Model file for the job. Use its own axes, mm. Face numbers are marked on the shaded views. A direction names the side the tool comes from. Round coordinates to 2 decimals unless told otherwise and drop trailing zeros. Loops run counter-clockwise (first coordinate to the right, second up) from the corner with the lowest first, then second, coordinate; pieces in that order, holes last. Notation, with made-up numbers: M 8.5,-29.75 L 52.5,-29.75 A8 cw 52.5,-19.75 Z; hole C 80.25,54 d4. An arc over 180 degrees is marked long. Use a Markdown table: item, result. Add a question column.
Item 1: Wall check: L1, parallel to Z at x = 6.5, y = -2; L2, parallel to Z at x = 5.25, y = 2.5; L3, parallel to Y at x = 5, z = 0.25. Give the ranges that are in metal, low to high. Write a range as from..to.
Item 2: Saw through at A-A on y = -0.25. Write the cut outline in (x, z), then the cut area to 3 significant figures.
Item 3: Pin check, flat tips, straight feed: P1, Ø0.7, axis at y = 3, z = 3.5, coming from the +X side; P2, Ø0.5, axis at x = 6, z = -5.5, coming from the +Y side; P3, Ø4, axis at y = -3.5, z = 0, coming from the -X side; P4, Ø1.2, axis at x = -6.5, y = -1.5, coming from the +Z side. Stop position of each tip, or through.
Item 4: Saw through at B-B on x = -2.25. Write the cut outline in (y, z).
Item 5: Saw through at C-C on z = -4.25. Write the cut outline in (x, y).
Item 6: Saw through at D-D on y = 2.25. Write the cut outline in (x, z), then the cut area to 3 significant figures.
Item 7: Two-plate mould, pull along X, no slides. Class the marked faces 4, 5 and 6: +X half, -X half, draft (parallel to the pull), parting line (faces both ways), or undercut.
Item 8: Tool access for the marked faces 1, 2 and 3: list every direction of +Z, -Z, +X, -X, +Y, -Y with a clear straight run to the whole face (end or side of a thin tool).
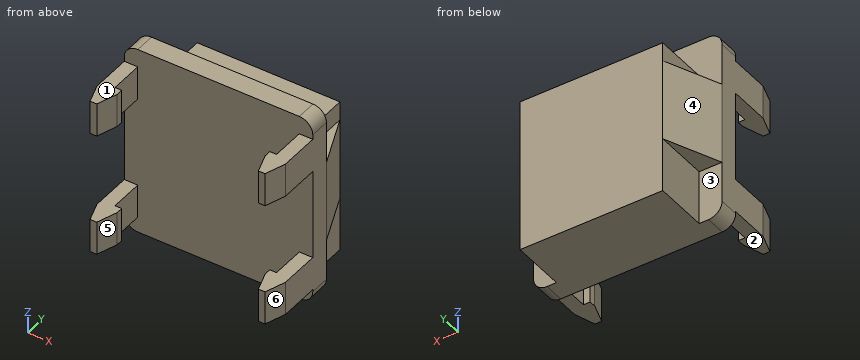
```python
from build123d import *

# Parameters (mm, degrees)
BOSS_EXTRUDE1_DEPTH = 1.5
SKETCH2_W           = 10.6
SKETCH2_H           = 11.5
BOSS_EXTRUDE2_DEPTH = 4
BOSS_EXTRUDE4_DEPTH = 6.07
SKETCH5_W           = 1.5
SKETCH5_H           = 2.5
BOSS_EXTRUDE5_DEPTH = 4.5
SKETCH6_W           = 0.5
SKETCH6_H           = 2.5
CUT_EXTRUDE1_DEPTH  = 16.632418239


with BuildPart() as part:
    # Sketch1 → Boss-Extrude1 (new body)
    with BuildSketch(Plane(origin=(0, 0, 0), x_dir=(1, 0, 0), z_dir=(0, 1, 0))):
        with BuildLine():
            Line((-6, -7.1), (6, -7.1))
            ThreePointArc((6, -7.1), (6.707106781, -6.807106781), (7, -6.1))
            Line((7, -6.1), (7, 6.1))
            ThreePointArc((7, 6.1), (6.707106781, 6.807106781), (6, 7.1))
            Line((6, 7.1), (-6, 7.1))
            ThreePointArc((-6, 7.1), (-6.707106781, 6.807106781), (-7, 6.1))
            Line((-7, 6.1), (-7, -6.1))
            ThreePointArc((-7, -6.1), (-6.707106781, -6.807106781), (-6, -7.1))
        make_face()
    extrude(amount=BOSS_EXTRUDE1_DEPTH)

    # Sketch2 → Boss-Extrude2 (add)
    with BuildSketch(Plane(origin=(0, 1.5, 0), x_dir=(1, 0, 0), z_dir=(0, 1, 0))):
        with Locations((0, 1.35)):
            Rectangle(SKETCH2_W, SKETCH2_H)
    extrude(amount=BOSS_EXTRUDE2_DEPTH)

    # Sketch4 → Boss-Extrude4 (add)
    with BuildSketch(Plane.XY.offset(3)):
        Polygon((-5.3, 5.5), (-7, 1.5), (-5.3, 1.5), align=None)
        Polygon((5.3, 5.5), (7, 1.5), (5.3, 1.5), align=None)
    extrude(amount=-BOSS_EXTRUDE4_DEPTH)

    # Sketch5 → Boss-Extrude5 (add)
    with BuildSketch(Plane.XZ):
        with Locations((-6.25, 4.5)):
            Rectangle(SKETCH5_W, SKETCH5_H)
        with Locations((-6.25, -4.7)):
            Rectangle(SKETCH5_W, SKETCH5_H)
        with Locations((6.25, -4.7)):
            Rectangle(SKETCH5_W, SKETCH5_H)
        with Locations((6.25, 4.5)):
            Rectangle(SKETCH5_W, SKETCH5_H)
    extrude(amount=BOSS_EXTRUDE5_DEPTH)

    # Sketch6 → Cut-Extrude1 (cut, through all)
    with BuildSketch(Plane.XY.offset(5.75)):
        with Locations((-5.75, -1.25)):
            Rectangle(SKETCH6_W, SKETCH6_H)
        Polygon((-7, -4.5), (-7, -3), (-6.5, -4.5), align=None)
        Polygon((-5.5, -3), (-6, -4.5), (-5.5, -4.5), align=None)
        with Locations((5.75, -1.25)):
            Rectangle(SKETCH6_W, SKETCH6_H)
        Polygon((5.5, -3), (6, -4.5), (5.5, -4.5), align=None)
        Polygon((7, -4.5), (7, -3), (6.5, -4.5), align=None)
    extrude(amount=-CUT_EXTRUDE1_DEPTH, mode=Mode.SUBTRACT)


solid = part.part
```
Entries:
| question | item | result |
|---|---|---|
| 1 | L1 | -5.95..-3.45, 3.25..5.75 |
| 1 | L2 | -7.1..4.4 |
| 1 | L3 | 0..5.5 |
| 2 | outline | M -7,-5.95 L -6,-5.95 L -6,-3.45 L -7,-3.45 Z; M -7,3.25 L -6,3.25 L -6,5.75 L -7,5.75 Z; M 6,-5.95 L 7,-5.95 L 7,-3.45 L 6,-3.45 Z; M 6,3.25 L 7,3.25 L 7,5.75 L 6,5.75 Z |
| 2 | area | 10.0 mm2 |
| 3 | P1 | x = 5.3 |
| 3 | P2 | y = 1.5 |
| 3 | P3 | through |
| 3 | P4 | z = 5.75 |
| 4 | outline | M 0,-7.1 L 5.5,-7.1 L 5.5,4.4 L 1.5,4.4 L 1.5,7.1 L 0,7.1 Z |
| 5 | outline | M -7,-3 L -6.5,-4.5 L -6,-4.5 L -5.5,-3 L -5.5,-2.5 L -6,-2.5 L -6,0 L 6,0 L 6,-2.5 L 5.5,-2.5 L 5.5,-3 L 6,-4.5 L 6.5,-4.5 L 7,-3 L 7,1.5 L 5.3,1.5 L 5.3,5.5 L -5.3,5.5 L -5.3,1.5 L -7,1.5 Z |
| 6 | outline | M -6.68,-3.07 L -5.3,-3.07 L -5.3,-7.1 L 5.3,-7.1 L 5.3,-3.07 L 6.68,-3.07 L 6.68,3 L 5.3,3 L 5.3,4.4 L -5.3,4.4 L -5.3,3 L -6.68,3 Z |
| 6 | area | 139 mm2 |
| 7 | face 4 | -X half |
| 7 | face 5 | undercut |
| 7 | face 6 | +X half |
| 8 | face 1 | +Z, +X, -X, -Y |
| 8 | face 2 | -Z, +X, -X, -Y |
| 8 | face 3 | -Z, -X, +Y |
